The model under review builds one solid part; all positions refer to its coordinate system, in mm. Face numbers are marked on the shaded views. A direction names the side the tool comes from. Coordinates: 2 decimals unless noted, no trailing zeros. Loops run counter-clockwise (first coordinate to the right, second up) from the corner with the lowest first, then second, coordinate; pieces in that order, holes last. Notation, with made-up numbers: (46, 49) - (65, 49) arc R23 ccw to (65, 74) - close; hole circle Ø9 at (7.25, -7.5). An arc over 180 degrees is marked (long way). One line per item, written item: value. Start each with the question number.
1. For the marked faces 1 and 2, list the 3-axis set-ups (+Z, -Z, +X, -X, +Y, -Y) from which the entire face can be reached by the end or side of a thin tool; tool diameter is ignored.
2. We need section C-C, the plane y = 1.4. Give the boundary of the cut face in (x, z), then the cut area to 3 significant figures.
3. We need section A-A, the plane y = 2.7. Give the boundary of the cut face in (x, z), then the cut area to 3 significant figures.
4. Insertion check: P1, Ø1.6, axis at x = 0.5, z = 7, coming from the +Y side. The pin has a flat end and moves straight along its axis. Give the tip position at first contact, or say it passes through.
5. We need section D-D, the plane z = -7.25. Give the boundary of the cut face in (x, y), then the cut area to 3 significant figures.
6. Mouldability with a two-part tool opening along Z and no side actions: class the marked faces 3, 4, 5 and 6 as +Z half, -Z half, draft (parallel to the pull), parting line (faces both ways), or undercut.
7. To check wall thickness, follow line 1 (Z direction, x = 8, y = 2.1) (3 decimals); line 2 (Z direction, x = 5, y = 2.4); line 3 (Y direction, x = 4, z = -7.75). State the ranges of each line that lie inside material, in increasing order.
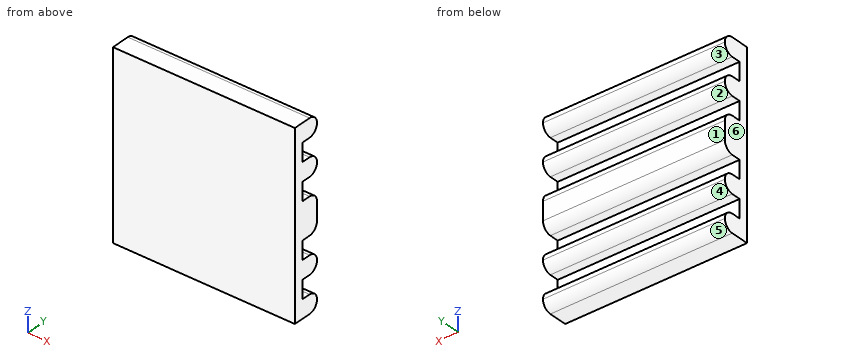
from build123d import *

# Parameters (mm, degrees)
SKETCH_1_W          = 20
SKETCH_1_H          = 20
EXTRUDE_1_DEPTH     = 3
SKETCH_2_W          = 20
SKETCH_2_H          = 2
CUT_EXTRUDE_1_DEPTH = 2
FILLET_1_R          = 1


with BuildPart() as part:
    # 草图1 → 凸台-拉伸1 (new body)
    with BuildSketch(Plane(origin=(0, 0, 0), x_dir=(1, 0, 0), z_dir=(0, 1, 0))):
        Rectangle(SKETCH_1_W, SKETCH_1_H)
    extrude(amount=EXTRUDE_1_DEPTH)

    # 草图2 → 切除-拉伸1 (cut)
    with BuildSketch(Plane(origin=(0, 3, 0), x_dir=(1, 0, 0), z_dir=(0, 1, 0))):
        with Locations((0, -7)):
            Rectangle(SKETCH_2_W, SKETCH_2_H)
        with Locations((0, -3)):
            Rectangle(SKETCH_2_W, SKETCH_2_H)
        with Locations((0, 7)):
            Rectangle(SKETCH_2_W, SKETCH_2_H)
        with Locations((0, 3)):
            Rectangle(SKETCH_2_W, SKETCH_2_H)
    extrude(amount=-CUT_EXTRUDE_1_DEPTH, mode=Mode.SUBTRACT)

    # 圆角1
    fillet_1_edges = [part.edges().sort_by_distance(p)[0] for p in [
        (0, 3, 10),
        (0, 3, 6),
        (0, 3, 8),
        (0, 3, -4),
        (0, 3, -2),
        (0, 3, -8),
        (0, 3, -6),
        (0, 3, 2),
        (0, 3, 4),
        (0, 3, -10),
    ]]
    fillet(fillet_1_edges, radius=FILLET_1_R - 0.0001)  # a hair under: the kernel refuses the full size


solid = part.part
Findings below:
1. face 1: +Z, -Z, +X, -X, +Y
1. face 2: +X, -X, +Y
2. outline: (-10, -10) - (10, -10) - (10, -8) - (-10, -8) - close; (-10, -6) - (10, -6) - (10, -4) - (-10, -4) - close; (-10, -2) - (10, -2) - (10, 2) - (-10, 2) - close; (-10, 4) - (10, 4) - (10, 6) - (-10, 6) - close; (-10, 8) - (10, 8) - (10, 10) - (-10, 10) - close
2. area: 240 mm2
3. outline: (-10, -9.71) - (10, -9.71) - (10, -8.29) - (-10, -8.29) - close; (-10, -5.71) - (10, -5.71) - (10, -4.29) - (-10, -4.29) - close; (-10, -1.71) - (10, -1.71) - (10, 1.71) - (-10, 1.71) - close; (-10, 4.29) - (10, 4.29) - (10, 5.71) - (-10, 5.71) - close; (-10, 8.29) - (10, 8.29) - (10, 9.71) - (-10, 9.71) - close
3. area: 183 mm2
4. P1: y = 1
5. outline: (-10, 0) - (10, 0) - (10, 1) - (-10, 1) - close
5. area: 20.0 mm2
6. face 3: undercut
6. face 4: undercut
6. face 5: -Z half
6. face 6: draft
7. line 1: -9.995 to -8.005, -5.995 to -4.005, -1.995 to 1.995, 4.005 to 5.995, 8.005 to 9.995
7. line 2: -9.92 to -8.08, -5.92 to -4.08, -1.92 to 1.92, 4.08 to 5.92, 8.08 to 9.92
7. line 3: 0 to 1
